Check sheet for the modelled part. Datum: model origin and axes. Units: mm. Give positions to 0.01 mm unless a question says otherwise; leave off trailing zeros. Order: outer loops, then holes, each group sorted by start corner. A loop starts at its lowest first (then second) coordinate and runs counter-clockwise, first axis right, second up. Notation, with made-up numbers: (15.5, -23.5) -> (53.5, -23.5) arc R27 ccw to (53.5, 1.5) -> close; hole circle Ø7 at (-33.5, -34). An arc over 180 degrees is marked (long way). Answer in a Markdown table with one row per item. Add a question column.
(1) Cross-section at A-A (y = -21). Record the cut outline in (x, z), then the cut area to 3 significant figures.
(2) Cross-section at B-B (x = -21). Record the cut outline in (y, z), then the cut area to 3 significant figures.
(3) Cross-section at C-C (x = 3). Record the cut outline in (y, z), then the cut area to 3 significant figures.
(4) Thickness scan on L1, parallel to X at y = -10, z = 1.1; L2, parallel to X at y = -23.5, z = 1.75; L3, parallel to Y at x = -11.5, z = 2.8. Record the ranges inside material, lowest first. Write a range as [from, to].
(5) Go/stop test with flat-tipped pins: pin 1 (0.9 mm diameter, centred on y = -24.5, z = 1, fed in from -X); pin 2 (1.5 mm diameter, centred on y = 22, z = 1.5, fed in from +X). Record where each tip stops, or that it passes through.
(6) Cross-section at D-D (x = 11.5). Record the cut outline in (y, z), then the cut area to 3 significant figures.
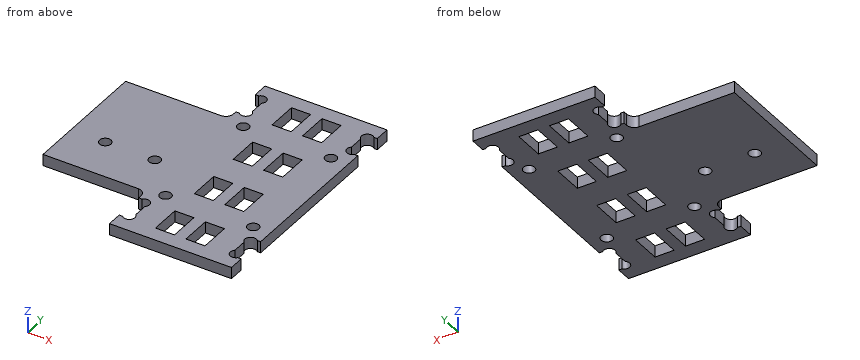
```python
from build123d import *

# Parameters (mm, degrees)
SKETCH_1_W                = 32
SKETCH_1_H                = 64
EXTRUDE_1_DEPTH           = 3
SKETCH_2_W                = 2.5
SKETCH_2_H                = 4
CUT_EXTRUDE_1_DEPTH       = 36.902646142
MIRROR_2_COPY_1_SKETCH_W  = 2.5
MIRROR_2_COPY_1_SKETCH_H  = 4
MIRROR_2_COPY_1_DEPTH     = 36.902646142
SKETCH_4_W                = 3
SKETCH_4_H                = 8
CUT_EXTRUDE_3_DEPTH       = 36.902646142
MIRROR_6_COPY_1_SKETCH_W  = 3
MIRROR_6_COPY_1_SKETCH_H  = 8
MIRROR_6_COPY_1_DEPTH     = 36.902646142
SKETCH_6_W                = 3
SKETCH_6_H                = 8
CUT_EXTRUDE_4_DEPTH       = 36.902646142
MIRROR_8_COPY_1_SKETCH_W  = 3
MIRROR_8_COPY_1_SKETCH_H  = 8
MIRROR_8_COPY_1_DEPTH     = 36.902646142
SKETCH_7_R                = 1.5
CUT_EXTRUDE_5_DEPTH       = 36.902646142
MIRROR_10_COPY_1_SKETCH_R = 1.5
MIRROR_10_COPY_1_DEPTH    = 36.902646142
SKETCH_8_R                = 1.5
CUT_EXTRUDE_6_DEPTH       = 36.902646142
MIRROR_12_COPY_1_SKETCH_R = 1.5
MIRROR_12_COPY_1_DEPTH    = 36.902646142
SKETCH_11_R               = 1.5
CUT_EXTRUDE_9_DEPTH       = 36.902646142
MIRROR_16_COPY_1_SKETCH_R = 1.5
MIRROR_16_COPY_1_DEPTH    = 36.902646142
SKETCH_12_W               = 5
SKETCH_12_H               = 8
CUT_EXTRUDE_10_DEPTH      = 36.902646142
MIRROR_18_COPY_1_SKETCH_W = 5
MIRROR_18_COPY_1_SKETCH_H = 8
MIRROR_18_COPY_1_DEPTH    = 36.902646142
SKETCH_13_W               = 3.954651238
SKETCH_13_H               = 10.848263898
SKETCH_13_W_2             = 4.227382692
SKETCH_13_H_2             = 10.655405874
EXTRUDE_2_DEPTH           = 3
SKETCH_14_W               = 27
SKETCH_14_H               = 34
EXTRUDE_3_DEPTH           = 3
SKETCH_15_R               = 1.5
CUT_EXTRUDE_11_DEPTH      = 54.684262126
FILLET_1_R                = 2


with BuildPart() as part:
    # 草图1 → 凸台-拉伸1 (new body)
    with BuildSketch(Plane.XY):
        Rectangle(SKETCH_1_W, SKETCH_1_H)
    extrude(amount=EXTRUDE_1_DEPTH)

    # 草图2 → 切除-拉伸1 (cut, through all)
    with BuildSketch(Plane.XY.offset(3)):
        Polygon((4, 8), (4, 4), (6.5, 4), (6.5, 12), (1.5, 12), (1.5, 8), align=None)
        with Locations((2.75, 6)):
            Rectangle(SKETCH_2_W, SKETCH_2_H)
    cut_extrude_1 = extrude(amount=-CUT_EXTRUDE_1_DEPTH, mode=Mode.SUBTRACT)

    # 镜向1: 切除-拉伸1 across plane
    add(cut_extrude_1.mirror(Plane(origin=(0, 0, 0), x_dir=(0, 0, 1), z_dir=(1, 0, 0))), mode=Mode.SUBTRACT)

    # 镜向2: 切除-拉伸1 across plane
    add(cut_extrude_1.mirror(Plane.ZX), mode=Mode.SUBTRACT)

    # 镜向2 copy 1 sketch → 镜向2 copy 1 (cut, through all)
    with BuildSketch(Plane(origin=(0, 0, 3), x_dir=(-1, 0, 0), z_dir=(0, 0, 1))):
        Polygon((4, 8), (4, 4), (6.5, 4), (6.5, 12), (1.5, 12), (1.5, 8), align=None)
        with Locations((2.75, 6)):
            Rectangle(MIRROR_2_COPY_1_SKETCH_W, MIRROR_2_COPY_1_SKETCH_H)
    extrude(amount=-MIRROR_2_COPY_1_DEPTH, mode=Mode.SUBTRACT)

    # 草图4 → 切除-拉伸3 (cut, through all)
    with BuildSketch(Plane.XY.offset(3)):
        with Locations((14.5, 8)):
            Rectangle(SKETCH_4_W, SKETCH_4_H)
    cut_extrude_3 = extrude(amount=-CUT_EXTRUDE_3_DEPTH, mode=Mode.SUBTRACT)

    # 镜向5: 切除-拉伸3 across plane
    add(cut_extrude_3.mirror(Plane(origin=(0, 0, 0), x_dir=(0, 0, 1), z_dir=(1, 0, 0))), mode=Mode.SUBTRACT)

    # 镜向6: 切除-拉伸3 across plane
    add(cut_extrude_3.mirror(Plane.ZX), mode=Mode.SUBTRACT)

    # 镜向6 copy 1 sketch → 镜向6 copy 1 (cut, through all)
    with BuildSketch(Plane(origin=(0, 0, 3), x_dir=(-1, 0, 0), z_dir=(0, 0, 1))):
        with Locations((14.5, 8)):
            Rectangle(MIRROR_6_COPY_1_SKETCH_W, MIRROR_6_COPY_1_SKETCH_H)
    extrude(amount=-MIRROR_6_COPY_1_DEPTH, mode=Mode.SUBTRACT)

    # 草图6 → 切除-拉伸4 (cut, through all)
    with BuildSketch(Plane.XY.offset(3)):
        with Locations((14.5, 24)):
            Rectangle(SKETCH_6_W, SKETCH_6_H)
    cut_extrude_4 = extrude(amount=-CUT_EXTRUDE_4_DEPTH, mode=Mode.SUBTRACT)

    # 镜向7: 切除-拉伸4 across plane
    add(cut_extrude_4.mirror(Plane(origin=(0, 0, 0), x_dir=(0, 0, 1), z_dir=(1, 0, 0))), mode=Mode.SUBTRACT)

    # 镜向8: 切除-拉伸4 across plane
    add(cut_extrude_4.mirror(Plane.ZX), mode=Mode.SUBTRACT)

    # 镜向8 copy 1 sketch → 镜向8 copy 1 (cut, through all)
    with BuildSketch(Plane(origin=(0, 0, 3), x_dir=(-1, 0, 0), z_dir=(0, 0, 1))):
        with Locations((14.5, 24)):
            Rectangle(MIRROR_8_COPY_1_SKETCH_W, MIRROR_8_COPY_1_SKETCH_H)
    extrude(amount=-MIRROR_8_COPY_1_DEPTH, mode=Mode.SUBTRACT)

    # 草图7 → 切除-拉伸5 (cut, through all)
    with BuildSketch(Plane.XY.offset(3)):
        with Locations((-14, 27)):
            Circle(SKETCH_7_R)
        with Locations((-14, 21)):
            Circle(SKETCH_7_R)
    cut_extrude_5 = extrude(amount=-CUT_EXTRUDE_5_DEPTH, mode=Mode.SUBTRACT)

    # 镜向9: 切除-拉伸5 across plane
    add(cut_extrude_5.mirror(Plane(origin=(0, 0, 0), x_dir=(0, 0, 1), z_dir=(1, 0, 0))), mode=Mode.SUBTRACT)

    # 镜向10: 切除-拉伸5 across plane
    add(cut_extrude_5.mirror(Plane.ZX), mode=Mode.SUBTRACT)

    # 镜向10 copy 1 sketch → 镜向10 copy 1 (cut, through all)
    with BuildSketch(Plane(origin=(0, 0, 3), x_dir=(-1, 0, 0), z_dir=(0, 0, 1))):
        with Locations((-14, 27)):
            Circle(MIRROR_10_COPY_1_SKETCH_R)
        with Locations((-14, 21)):
            Circle(MIRROR_10_COPY_1_SKETCH_R)
    extrude(amount=-MIRROR_10_COPY_1_DEPTH, mode=Mode.SUBTRACT)

    # 草图8 → 切除-拉伸6 (cut, through all)
    with BuildSketch(Plane.XY.offset(3)):
        with Locations((-14, 11)):
            Circle(SKETCH_8_R)
        with Locations((-14, 5)):
            Circle(SKETCH_8_R)
    cut_extrude_6 = extrude(amount=-CUT_EXTRUDE_6_DEPTH, mode=Mode.SUBTRACT)

    # 镜向11: 切除-拉伸6 across plane
    add(cut_extrude_6.mirror(Plane(origin=(0, 0, 0), x_dir=(0, 0, 1), z_dir=(1, 0, 0))), mode=Mode.SUBTRACT)

    # 镜向12: 切除-拉伸6 across plane
    add(cut_extrude_6.mirror(Plane.ZX), mode=Mode.SUBTRACT)

    # 镜向12 copy 1 sketch → 镜向12 copy 1 (cut, through all)
    with BuildSketch(Plane(origin=(0, 0, 3), x_dir=(-1, 0, 0), z_dir=(0, 0, 1))):
        with Locations((-14, 11)):
            Circle(MIRROR_12_COPY_1_SKETCH_R)
        with Locations((-14, 5)):
            Circle(MIRROR_12_COPY_1_SKETCH_R)
    extrude(amount=-MIRROR_12_COPY_1_DEPTH, mode=Mode.SUBTRACT)

    # 草图11 → 切除-拉伸9 (cut, through all)
    with BuildSketch(Plane.XY.offset(3)):
        with Locations((11.5, 16)):
            Circle(SKETCH_11_R)
    cut_extrude_9 = extrude(amount=-CUT_EXTRUDE_9_DEPTH, mode=Mode.SUBTRACT)

    # 镜向15: 切除-拉伸9 across plane
    add(cut_extrude_9.mirror(Plane(origin=(0, 0, 0), x_dir=(0, 0, 1), z_dir=(1, 0, 0))), mode=Mode.SUBTRACT)

    # 镜向16: 切除-拉伸9 across plane
    add(cut_extrude_9.mirror(Plane.ZX), mode=Mode.SUBTRACT)

    # 镜向16 copy 1 sketch → 镜向16 copy 1 (cut, through all)
    with BuildSketch(Plane(origin=(0, 0, 3), x_dir=(-1, 0, 0), z_dir=(0, 0, 1))):
        with Locations((11.5, 16)):
            Circle(MIRROR_16_COPY_1_SKETCH_R)
    extrude(amount=-MIRROR_16_COPY_1_DEPTH, mode=Mode.SUBTRACT)

    # 草图12 → 切除-拉伸10 (cut, through all)
    with BuildSketch(Plane.XY.offset(3)):
        with Locations((4, 24)):
            Rectangle(SKETCH_12_W, SKETCH_12_H)
    cut_extrude_10 = extrude(amount=-CUT_EXTRUDE_10_DEPTH, mode=Mode.SUBTRACT)

    # 镜向17: 切除-拉伸10 across plane
    add(cut_extrude_10.mirror(Plane(origin=(0, 0, 0), x_dir=(0, 0, 1), z_dir=(1, 0, 0))), mode=Mode.SUBTRACT)

    # 镜向18: 切除-拉伸10 across plane
    add(cut_extrude_10.mirror(Plane.ZX), mode=Mode.SUBTRACT)

    # 镜向18 copy 1 sketch → 镜向18 copy 1 (cut, through all)
    with BuildSketch(Plane(origin=(0, 0, 3), x_dir=(-1, 0, 0), z_dir=(0, 0, 1))):
        with Locations((4, 24)):
            Rectangle(MIRROR_18_COPY_1_SKETCH_W, MIRROR_18_COPY_1_SKETCH_H)
    extrude(amount=-MIRROR_18_COPY_1_DEPTH, mode=Mode.SUBTRACT)

    # 草图13 → 凸台-拉伸2 (add)
    with BuildSketch(Plane.XY.offset(3)):
        with Locations((-14.022674381, 8.035470268)):
            Rectangle(SKETCH_13_W, SKETCH_13_H)
        with Locations((13.886308654, 8.035470268)):
            Rectangle(SKETCH_13_W_2, SKETCH_13_H)
        with Locations((13.886308654, -7.875316782)):
            Rectangle(SKETCH_13_W_2, SKETCH_13_H_2)
        with Locations((-14.022674381, -7.875316782)):
            Rectangle(SKETCH_13_W, SKETCH_13_H_2)
    extrude(amount=-EXTRUDE_2_DEPTH)

    # 草图14 → 凸台-拉伸3 (add)
    with BuildSketch(Plane(origin=(0, 0, 0), x_dir=(-1, 0, 0), z_dir=(0, 0, -1))):
        with Locations((29.5, 0)):
            Rectangle(SKETCH_14_W, SKETCH_14_H)
    extrude(amount=-EXTRUDE_3_DEPTH)

    # 草图15 → 切除-拉伸11 (cut, through all)
    with BuildSketch(Plane(origin=(0, 0, 0), x_dir=(-1, 0, 0), z_dir=(0, 0, -1))):
        with Locations((34, -5.5)):
            Circle(SKETCH_15_R)
        with Locations((21, -5.5)):
            Circle(SKETCH_15_R)
    extrude(amount=-CUT_EXTRUDE_11_DEPTH, mode=Mode.SUBTRACT)

    # 圆角1
    fillet_1_edges = [part.edges().sort_by_distance(p)[0] for p in [
        (-16, -17, 1.5),
        (-16, 17, 1.5),
    ]]
    fillet(fillet_1_edges, radius=FILLET_1_R)


solid = part.part
```
Answer below:
| question | item | result |
|---|---|---|
| 1 | outline | (-12.5, 0) -> (-6.5, 0) -> (-6.5, 3) -> (-12.5, 3) -> close; (-1.5, 0) -> (1.5, 0) -> (1.5, 3) -> (-1.5, 3) -> close; (6.5, 0) -> (12.5, 0) -> (12.5, 3) -> (6.5, 3) -> close |
| 1 | area | 45.0 mm² |
| 2 | outline | (-17, 0) -> (-7, 0) -> (-7, 3) -> (-17, 3) -> close; (-4, 0) -> (17, 0) -> (17, 3) -> (-4, 3) -> close |
| 2 | area | 93.0 mm² |
| 3 | outline | (-32, 0) -> (-28, 0) -> (-28, 3) -> (-32, 3) -> close; (-20, 0) -> (-12, 0) -> (-12, 3) -> (-20, 3) -> close; (-4, 0) -> (4, 0) -> (4, 3) -> (-4, 3) -> close; (12, 0) -> (20, 0) -> (20, 3) -> (12, 3) -> close; (28, 0) -> (32, 0) -> (32, 3) -> (28, 3) -> close |
| 3 | area | 96.0 mm² |
| 4 | L1 | x = [-43, -6.5], [-1.5, 1.5], [6.5, 16] |
| 4 | L2 | x = [-13, -6.5], [-1.5, 1.5], [6.5, 13] |
| 4 | L3 | y = [-32, -17.5], [-14.5, 14.5], [17.5, 32] |
| 5 | pin 1 | stops at x = -13 |
| 5 | pin 2 | stops at x = 13 |
| 6 | outline | (-32, 0) -> (-17.5, 0) -> (-17.5, 3) -> (-32, 3) -> close; (-14.5, 0) -> (14.5, 0) -> (14.5, 3) -> (-14.5, 3) -> close; (17.5, 0) -> (32, 0) -> (32, 3) -> (17.5, 3) -> close |
| 6 | area | 174 mm² |
